Design review of the part built by this model. Coordinates are the model's own, in mm. Face numbers are marked on the shaded views. A direction names the side the tool comes from. Round coordinates to 2 decimals unless told otherwise and drop trailing zeros. Loops run counter-clockwise (first coordinate to the right, second up) from the corner with the lowest first, then second, coordinate; pieces in that order, holes last. Notation, with made-up numbers: (50, 39) - (90, 39) arc R20 cw to (90, 46) - close; hole circle Ø3 at (-7, 25.5). An arc over 180 degrees is marked (long way). Use one line per item in the form item = value. Start each with the question number.
(1) We need section C-C, the plane y = 12. Write out the cut boundary in (x, z), then the cut area to 3 significant figures.
(2) We need section B-B, the plane z = -63. Write out the cut boundary in (x, y) (3 decimals).
(3) Wall thickness on probe 1 along Y at (x, z) = (12.75, -23) (3 decimals); probe 2 along Y at (x, z) = (-1.5, -90); probe 3 along Z at (x, y) = (0, -1.5): over which ranges is each line inside the solid? List them lowest first. Write a range as [from, to].
(4) The part is to be moulded in two halves that separate along Z. For the marked faces 1, 2, 3 and 4, say which applies: released by +Z, released by -Z, zero draft, split by the parting line, or undercut.
(5) For pin 1 (3 mm diameter, centred on x = 8.5, y = 11.5, fed in from +Z); pin 2 (6 mm diameter, centred on x = 4, y = 16.5, fed in from -Z); pin 3 (4 mm diameter, centred on y = -21, z = 53.5, fed in from -X); pin 4 (5 mm diameter, centred on x = 12, y = 20.5, fed in from -Z), all flat-tipped, find the tip position at first contact; note any pin that passes through.
(6) We need section A-A, the plane x = 3.5. Write out the cut boundary in (y, z) (3 decimals), then the cut area to 3 significant figures.
(7) Machinability: for the marked faces 5 and 6, which of the approach directions +Z, -Z, +X, -X, +Y, -Y give a long, thin tool a straight path to every point of the face, cutting with its end or side? Answer none if there is none.
from build123d import *

# Parameters (mm, degrees)
EXTRUDE_1_DEPTH      = 15
EXTRUDE_1_DEPTH_BACK = 15
CUT_EXTRUDE_1_DEPTH  = 30


with BuildPart() as part:
    # Sketch 2 → Extrude 1 (new body, two sides)
    with BuildSketch(Plane(origin=(0, 0, 0), x_dir=(0, 0, -1), z_dir=(1, 0, 0))) as extrude_1_sk:
        with BuildLine():
            Line((-76, 27.345), (76, 27.345))
            ThreePointArc((76, 27.345), (103.345, 0), (76, -27.345))
            Line((76, -27.345), (-76, -27.345))
            ThreePointArc((-76, -27.345), (-103.345, 0), (-76, 27.345))
        make_face()
    extrude(amount=EXTRUDE_1_DEPTH)
    extrude(extrude_1_sk.sketch, amount=-EXTRUDE_1_DEPTH_BACK)

    # Sketch 3 → Cut-Extrude 1 (cut)
    with BuildSketch(Plane(origin=(15, 0, 0), x_dir=(0, 0, -1), z_dir=(1, 0, 0))):
        with BuildLine():
            Line((-76, 21.345), (76, 21.345))
            ThreePointArc((76, 21.345), (97.345, 0), (76, -21.345))
            Line((76, -21.345), (-76, -21.345))
            ThreePointArc((-76, -21.345), (-97.345, 0), (-76, 21.345))
        make_face()
    extrude(amount=-CUT_EXTRUDE_1_DEPTH, mode=Mode.SUBTRACT)


solid = part.part
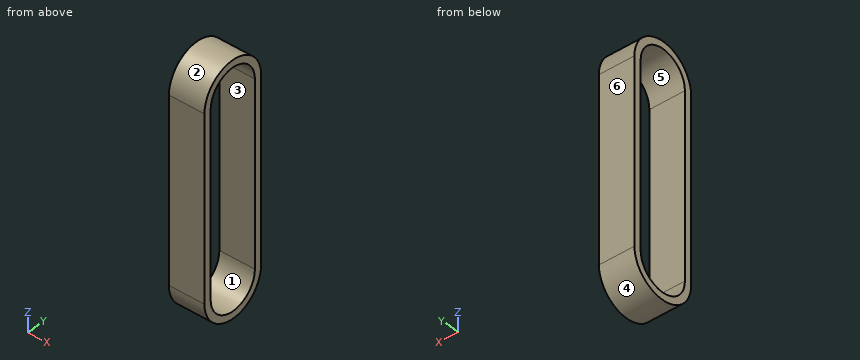
Data:
q1.outline = (-15, -100.57) - (15, -100.57) - (15, -93.65) - (-15, -93.65) - close; (-15, 93.65) - (15, 93.65) - (15, 100.57) - (-15, 100.57) - close
q1.area = 415 mm^2
q2.outline = (-15, -27.345) - (15, -27.345) - (15, -21.345) - (-15, -21.345) - close; (-15, 21.345) - (15, 21.345) - (15, 27.345) - (-15, 27.345) - close
q3.probe_1 = [-27.345, -21.345], [21.345, 27.345]
q3.probe_2 = [-23.49, -16.11], [16.11, 23.49]
q3.probe_3 = [-103.3, -97.29], [97.29, 103.3]
q4.face_1 = undercut
q4.face_2 = released by +Z
q4.face_3 = undercut
q4.face_4 = released by -Z
q5.pin_1 = 101.45
q5.pin_2 = -99.78
q5.pin_3 = -15
q5.pin_4 = -96.59
q6.outline = (-27.345, -76) arc R27.345 ccw to (27.345, -76) - (27.345, 76) arc R27.345 ccw to (-27.345, 76) - close; hole (-21.345, -76) arc R21.345 ccw to (21.345, -76) - (21.345, 76) arc R21.345 ccw to (-21.345, 76) - close
q6.area = 2,740 mm^2
q7.face_5 = +X, -X
q7.face_6 = +Z, -Z, +X, -X, +Y
